from build123d import *

# Parameters (mm, degrees)
EXTRUDE_1_DEPTH     = 5
SKETCH_2_R          = 2
CUT_EXTRUDE_1_DEPTH = 6


with BuildPart() as part:
    # 草图1 → 凸台-拉伸1 (new body)
    with BuildSketch(Plane.XY):
        with BuildLine():
            Line((-52, 12.5), (52, 12.5))
            ThreePointArc((52, 12.5), (54.121320344, 11.621320344), (55, 9.5))
            Line((55, 9.5), (55, -9.5))
            ThreePointArc((55, -9.5), (54.121320344, -11.621320344), (52, -12.5))
            Line((52, -12.5), (-52, -12.5))
            ThreePointArc((-52, -12.5), (-54.121320344, -11.621320344), (-55, -9.5))
            Line((-55, -9.5), (-55, 9.5))
            ThreePointArc((-55, 9.5), (-54.121320344, 11.621320344), (-52, 12.5))
        make_face()
    extrude(amount=-EXTRUDE_1_DEPTH)

    # 草图2 → 切除-拉伸1 (cut, through all)
    with BuildSketch(Plane.XY):
        with Locations((50, 0)):
            Circle(SKETCH_2_R)
        with Locations((-50, 0)):
            Circle(SKETCH_2_R)
    extrude(amount=-CUT_EXTRUDE_1_DEPTH, mode=Mode.SUBTRACT)


solid = part.part
Design review of the part built by this model. Coordinates are the model's own, in mm. Coordinates: 2 decimals unless noted, no trailing zeros. Loops run counter-clockwise (first coordinate to the right, second up) from the corner with the lowest first, then second, coordinate; pieces in that order, holes last.
Item 1: Clearance check with a flat-ended pin moving along its axis: pin 1 (4.5 mm diameter, centred on x = 50, y = 0, fed in from -Z). State where the tip first meets the part, or that it passes through.
Completed:
pin 1: stops at z = -5
Item 2: Add section A-A (y = 0). Write out the cut boundary in (x, z), and give its area (3 significant figures).
Completed:
outline: (-55, -5) - (-52, -5) - (-52, 0) - (-55, 0) - close; (-48, -5) - (48, -5) - (48, 0) - (-48, 0) - close; (52, -5) - (55, -5) - (55, 0) - (52, 0) - close
area: 510 mm2
Item 3: Wall thickness on L1, parallel to Y at x = 50, z = -1.4; L2, parallel to X at y = 0.75, z = -2.2; L3, parallel to X at y = 11, z = -3: over which ranges is each line inside the solid? List them lowest first.
Completed:
L1: y = -12.5 to -2, 2 to 12.5
L2: x = -55 to -51.85, -48.15 to 48.15, 51.85 to 55
L3: x = -54.6 to 54.6
Item 4: Draft analysis for pull direction X (two halves, no side actions). For faces 1 (the flat face through (1, -12.5, -2)), 2 (the cylindrical face through (-52, 0, -2)), 3 (the cylindrical face through (-54.14, 11.6, -2.46)), state which applies: pulls with the +X half, pulls with the -X half, needs draft (parallel to the pull), parting line crosses it, or undercut.
Completed:
face 1: needs draft
face 2: undercut
face 3: pulls with the -X half
Item 5: Add section B-B (x = -50). Write out the cut boundary in (y, z), and give its area (3 significant figures).
Completed:
outline: (-12.5, -5) - (-2, -5) - (-2, 0) - (-12.5, 0) - close; (2, -5) - (12.5, -5) - (12.5, 0) - (2, 0) - close
area: 105 mm2
